from build123d import *

# Parameters (mm, degrees)
SKETCH_W        = 100
SKETCH_H        = 50
PAD_DEPTH       = 30
SKETCH002_W     = 20
SKETCH002_H     = 30
POCKET_DEPTH    = 30
SKETCH003_W     = 20
SKETCH003_H     = 30
POCKET001_DEPTH = 30
SKETCH004_W     = 20
SKETCH004_H     = 30
POCKET002_DEPTH = 30
SKETCH005_R     = 5
POCKET003_DEPTH = 18


with BuildPart() as part:
    # Sketch → Pad (new body)
    with BuildSketch(Plane.XY):
        with Locations((-20.333326, 4.957771)):
            Rectangle(SKETCH_W, SKETCH_H)
    extrude(amount=PAD_DEPTH)

    # Sketch002 (on Face6 of Pad) → Pocket (cut)
    with BuildSketch(Plane.XY.offset(30)):
        with Locations((-50.136953, 4.881032)):
            Rectangle(SKETCH002_W, SKETCH002_H)
    extrude(amount=-POCKET_DEPTH, mode=Mode.SUBTRACT)

    # Sketch003 (on Face5 of Pocket) → Pocket001 (cut)
    with BuildSketch(Plane.XY.offset(30)):
        with Locations((-20.07695, 5.053894)):
            Rectangle(SKETCH003_W, SKETCH003_H)
    extrude(amount=-POCKET001_DEPTH, mode=Mode.SUBTRACT)

    # Sketch004 (on Face5 of Pocket001) → Pocket002 (cut)
    with BuildSketch(Plane.XY.offset(30)):
        with Locations((10, 4.949642)):
            Rectangle(SKETCH004_W, SKETCH004_H)
    extrude(amount=-POCKET002_DEPTH, mode=Mode.SUBTRACT)

    # Sketch005 (on Face1 of Pocket002) → Pocket003 (cut)
    with BuildSketch(Plane(origin=(-70.333326, 0, 0), x_dir=(0, -1, 0), z_dir=(-1, 0, 0))):
        with Locations((-5.017015, 14.892237)):
            Circle(SKETCH005_R)
    extrude(amount=-POCKET003_DEPTH, mode=Mode.SUBTRACT)


solid = part.part
Can you work these out from the model? Positions are in its coordinate system, mm. A direction names the side the tool comes from. Round coordinates to 2 decimals unless told otherwise and drop trailing zeros. Loops run counter-clockwise (first coordinate to the right, second up) from the corner with the lowest first, then second, coordinate; pieces in that order, holes last. Notation, with made-up numbers: (-25, -40) - (1, -40) arc R35 ccw to (1, -6) - close; hole circle Ø11 at (86, 2.5). An arc over 180 degrees is marked (long way). Use CSV: the item, a comma, the result in double quotes. Start each with the question number.
1) Please list where these lines run through material, in increasing order: probe 1 along X at (y, z) = (2, 12); probe 2 along X at (y, z) = (-7, 11.5); probe 3 along Y at (x, z) = (-56.5, 12.75). Write a range as [from, to].
2) If we section it at B-B on x = 5: Write out the boundary of the cut face in (y, z).
3) If we section it at D-D on y = 8.5: Write out the boundary of the cut face in (x, z).
4) For pin 1 Ø1.5 at (x, y) = (-28.5, -0.5) entering from +Z, with a flat end and sliding along its axis, tell me the tip position at first contact or that it passes through.
5) For faces 1 (the flat face through (-21, 29.958, 15)), 2 (the flat face through (-50, 19.881, 15)), which set-ups out of +Z, -Z, +X, -X, +Y, -Y let a thin tool reach every point of the face, with its end or its side?
6) If we section it at C-C on z = 21: Write out the boundary of the cut face in (x, y), plus the area to 3 significant figures.
7) We'd pull the mould along Z, two halves only. Please class faces 3 (the cylindrical face through (-65.31, 6.1, 10.01)), 4 (the flat face through (-32, 5, 30)), 5 (the flat face through (20, 5, 15)): released by +Z, released by -Z, zero draft, split by the parting line, or undercut.
8) If we section it at A-A on y = -2: Write out the boundary of the cut face in (x, z), plus the area to 3 significant figures.
Geometry results:
1,probe 1,"x = [-40.14, -30.08], [-10.08, 0], [20, 29.67]"
1,probe 2,"x = [-70.33, -60.14], [-40.14, -30.08], [-10.08, 0], [20, 29.67]"
1,probe 3,"y = [-20.04, -10.12], [19.88, 29.96]"
2,outline,"(-20.04, 0) - (-10.05, 0) - (-10.05, 30) - (-20.04, 30) - close; (19.95, 0) - (29.96, 0) - (29.96, 30) - (19.95, 30) - close"
3,outline,"(-70.33, 0) - (-60.14, 0) - (-60.14, 11.3) - (-70.33, 11.3) - close; (-70.33, 18.48) - (-60.14, 18.48) - (-60.14, 30) - (-70.33, 30) - close; (-40.14, 0) - (-30.08, 0) - (-30.08, 30) - (-40.14, 30) - close; (-10.08, 0) - (0, 0) - (0, 30) - (-10.08, 30) - close; (20, 0) - (29.67, 0) - (29.67, 30) - (20, 30) - close"
4,pin 1,"passes through"
5,face 1,"+Z, -Z, +X, -X, +Y"
5,face 2,"+Z, -Z"
6,outline,"(-70.33, -20.04) - (29.67, -20.04) - (29.67, 29.96) - (-70.33, 29.96) - close; hole (-60.14, -10.12) - (-40.14, -10.12) - (-40.14, 19.88) - (-60.14, 19.88) - close; hole (-30.08, -9.95) - (-10.08, -9.95) - (-10.08, 20.05) - (-30.08, 20.05) - close; hole (0, -10.05) - (20, -10.05) - (20, 19.95) - (0, 19.95) - close"
6,area,"3,200 mm2"
7,face 3,"undercut"
7,face 4,"released by +Z"
7,face 5,"zero draft"
8,outline,"(-70.33, 0) - (-60.14, 0) - (-60.14, 30) - (-70.33, 30) - close; (-40.14, 0) - (-30.08, 0) - (-30.08, 30) - (-40.14, 30) - close; (-10.08, 0) - (0, 0) - (0, 30) - (-10.08, 30) - close; (20, 0) - (29.67, 0) - (29.67, 30) - (20, 30) - close"
8,area,"1,200 mm2"
